Source: CAD feature listing. Evaluate the final solid. Frame: model axes, mm. Face numbers are marked on the shaded views. A direction names the side the tool comes from. Coordinates: 2 decimals unless noted, no trailing zeros. Loops run counter-clockwise (first coordinate to the right, second up) from the corner with the lowest first, then second, coordinate; pieces in that order, holes last.
Item 1: Section query B-B, the plane x = -102.5. Return the cut outline in (y, z) (3 decimals).
Item 2: Reachability of the marked faces 4 and 5 from +Z, -Z, +X, -X, +Y, -Y: full face, straight path, thin tool, end or side. Return the list, or none.
Item 3: Section query C-C, the plane y = 211. Return the cut outline in (x, z).
Item 4: Line query: probe 1 along X at (y, z) = (134, 41.5); probe 2 along Y at (x, z) = (19, 5) (3 decimals); probe 3 along Z at (x, y) = (-60.5, 202.5). Output: solid intervals per line, ascending.
Item 5: Section query A-A, the plane z = -33. Return the cut outline in (x, y) (3 decimals), then the cut area to 3 significant figures.
Item 6: Pull-direction query (X, two-part tool) for the marked faces 1, 2 and 3; classes: +X half, -X half, draft (parallel to the pull), parting line (faces both ways), or undercut.
Item 7: Pin query (flat end, axial travel): pin 1 Ø1.5 at (x, y) = (-9.5, 126.5) entering from +Z; pin 2 Ø1.7 at (x, y) = (-2.5, 376.5) entering from +Z. Return the tip coordinate at first contact, or that it passes through.
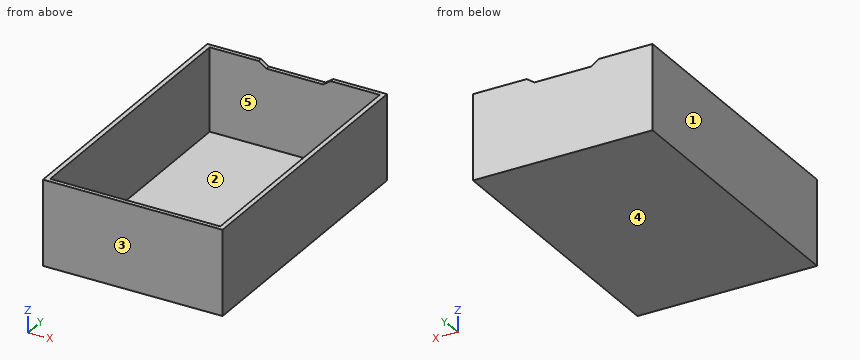
```python
from build123d import *

# Parameters (mm, degrees)
SKETCH1_W           = 241.3
SKETCH1_H           = 114.3
BOSS_EXTRUDE1_DEPTH = 379.73
SKETCH2_W           = 228.6
SKETCH2_H           = 368.3
CUT_EXTRUDE1_DEPTH  = 111.76
CUT_EXTRUDE2_DEPTH  = 111.76


with BuildPart() as part:
    # Sketch1 → Boss-Extrude1 (new body)
    with BuildSketch(Plane(origin=(0, 0, 0), x_dir=(1, 0, 0), z_dir=(0, 1, 0))):
        Rectangle(SKETCH1_W, SKETCH1_H)
    extrude(amount=BOSS_EXTRUDE1_DEPTH)

    # Sketch2 → Cut-Extrude1 (cut)
    with BuildSketch(Plane.XY.offset(57.15)):
        with Locations((0, 189.865)):
            Rectangle(SKETCH2_W, SKETCH2_H)
    extrude(amount=-CUT_EXTRUDE1_DEPTH, mode=Mode.SUBTRACT)

    # Sketch3 → Cut-Extrude2 (cut)
    with BuildSketch(Plane(origin=(0, 379.73, 0), x_dir=(1, 0, 0), z_dir=(0, 1, 0))):
        Polygon((-38.1, -49.883610426), (-48.510901929, -57.15), (48.384797494, -57.15), (38.1, -49.883610426), align=None)
    extrude(amount=-CUT_EXTRUDE2_DEPTH, mode=Mode.SUBTRACT)


solid = part.part
```
Verdict:
1. outline: (0, -57.15) - (379.73, -57.15) - (379.73, 57.15) - (374.015, 57.15) - (374.015, -54.61) - (5.715, -54.61) - (5.715, 57.15) - (0, 57.15) - close
2. face 4: -Z, +X, -X, +Y, -Y
2. face 5: +Z
3. outline: (-120.65, -57.15) - (120.65, -57.15) - (120.65, 57.15) - (114.3, 57.15) - (114.3, -54.61) - (-114.3, -54.61) - (-114.3, 57.15) - (-120.65, 57.15) - close
4. probe 1: x = -120.65 to -114.3, 114.3 to 120.65
4. probe 2: y = 0 to 5.715, 374.015 to 379.73
4. probe 3: z = -57.15 to -54.61
5. outline: (-120.65, 0) - (120.65, 0) - (120.65, 379.73) - (-120.65, 379.73) - close; hole (-114.3, 5.715) - (114.3, 5.715) - (114.3, 374.015) - (-114.3, 374.015) - close
5. area: 7,440 mm2
6. face 1: -X half
6. face 2: undercut
6. face 3: draft
7. pin 1: stops at z = -54.61
7. pin 2: stops at z = 49.88
